```python
from build123d import *

# Parameters (mm, degrees)
F0_W      = 37
F0_H      = 107
F1_DEPTH  = 1.5
F2_W      = 37
F2_H      = 107
F2_W_2    = 33
F2_H_2    = 103
F3_DEPTH  = 15
F4_W      = 7
F4_H      = 7
F5_DEPTH  = 5
F6_R      = 1.5
F7_DEPTH  = 5
F8_R      = 3
F9_W      = 8
F9_H      = 11.456422
F10_DEPTH = 25
F11_W     = 12
F11_H     = 3
F11_H_2   = 4
F11_W_2   = 10
F11_H_3   = 12.768078
F12_DEPTH = 25
F13_R     = 3


with BuildPart() as f1:
    # F0 (on Top) → F1 (new body)
    with BuildSketch(Plane.XY):
        Rectangle(F0_W, F0_H)
    extrude(amount=F1_DEPTH)

    # F2 (on face) → F3 (join)
    with BuildSketch(Plane.XY.offset(1.5)):
        Rectangle(F2_W, F2_H)
        Rectangle(F2_W_2, F2_H_2, mode=Mode.SUBTRACT)
    extrude(amount=F3_DEPTH)

    # F4 (on face) → F5 (join)
    with BuildSketch(Plane.XY.offset(1.5)):
        with Locations((-13, 48)):
            Rectangle(F4_W, F4_H)
        with Locations((13, 48)):
            Rectangle(F4_W, F4_H)
        with Locations((13, -48)):
            Rectangle(F4_W, F4_H)
        with Locations((-13, -48)):
            Rectangle(F4_W, F4_H)
    extrude(amount=F5_DEPTH)

    # F6 (on face) → F7 (cut)
    with BuildSketch(Plane.XY.offset(6.5)):
        with Locations((-12.5, 47.5)):
            Circle(F6_R)
        with Locations((12.5, 47.5)):
            Circle(F6_R)
        with Locations((12.5, -47.5)):
            Circle(F6_R)
        with Locations((-12.5, -47.5)):
            Circle(F6_R)
    extrude(amount=-F7_DEPTH, mode=Mode.SUBTRACT)

    # F8
    f8_edges = [f1.edges().sort_by_distance(p)[0] for p in [
        (-9.5, 44.5, 4),
        (9.5, 44.5, 4),
        (-9.5, -44.5, 4),
        (9.5, -44.5, 4),
    ]]
    fillet(f8_edges, radius=F8_R)

    # F9 (on face) → F10 (cut)
    with BuildSketch(Plane(origin=(0, -51.5, 0), x_dir=(-1, 0, 0), z_dir=(0, 1, 0))):
        with Locations((4, 12.228211)):
            Rectangle(F9_W, F9_H)
        with Locations((-4, 12.228211)):
            Rectangle(F9_W, F9_H)
    extrude(amount=-F10_DEPTH, mode=Mode.SUBTRACT)

    # F11 (on face) → F12 (cut)
    with BuildSketch(Plane(origin=(-18.5, 0, 0), x_dir=(0, -1, 0), z_dir=(-1, 0, 0))):
        with Locations((-39.5, 8)):
            Rectangle(F11_W, F11_H)
        with Locations((-39.5, 4.5)):
            Rectangle(F11_W, F11_H_2)
        with Locations((37.5, 12.884039)):
            Rectangle(F11_W_2, F11_H_3)
    extrude(amount=-F12_DEPTH, mode=Mode.SUBTRACT)

    # F13
    f13_edges = [f1.edges().sort_by_distance(p)[0] for p in [
        (18.5, -53.5, 8.25),
        (-18.5, -53.5, 8.25),
        (-18.5, 53.5, 8.25),
        (18.5, 53.5, 8.25),
    ]]
    fillet(f13_edges, radius=F13_R)


solid = f1.part
```
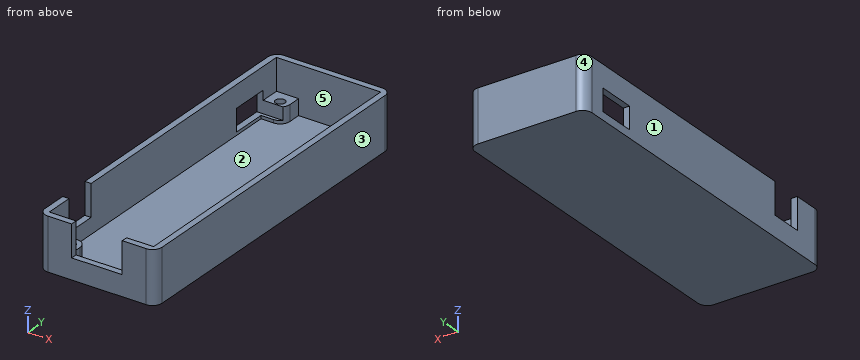
The listing builds one solid part. Answer for the finished solid, in the listing's coordinates (mm). Face numbers are marked on the shaded views. A direction names the side the tool comes from. Round coordinates to 2 decimals unless told otherwise and drop trailing zeros. Write each loop counter-clockwise with the first axis right and the second up, starting at its lowest first coordinate (ties: lowest second). Pieces come first, ordered by that corner, then holes. Notation, with made-up numbers: (-10, 13.5) -> (10, 13.5) arc R18 ccw to (10, 25.5) -> close; hole circle Ø7 at (-37.75, 73.25). An arc over 180 degrees is marked (long way). Answer as a JSON object with one key per item and string values. Group by question number.
Q1. Each of these flat-tipped pins is pushed along its axis until it touches: pin 1 Ø2 at (x, z) = (-18, 9.5) entering from +Y; pin 2 Ø6 at (x, y) = (3, -28.5) entering from +Z; pin 3 Ø6.5 at (x, y) = (-12, 47) entering from +Z. Where does it stop, or does it pass through?
Q2. Section A-A (y = 36) is taken. Write down the section's boundary in (x, z), plus the area to 4 significant figures.
Q3. Which of the six approach directions +Z, -Z, +X, -X, +Y, -Y give full straight-line access (tool end or side, diameter ignored) to the marked faces 4 and 5?
Q4. Straight lines are drawn through the part: line 1 along Y through (x, z) = (-12.5, 2.7); line 2 along Y through (x, z) = (12.5, 3.65); line 3 along X through (y, z) = (41.5, 15.75). For each, find the intervals that lie inside material, in ascending order.
Q5. Section C-C (y = 2.5) is taken. Write down the section's boundary in (x, z).
Q6. Section B-B (z = 12.75) is taken. Write down the section's boundary in (x, y).
Q7. Determine the mould class of the marked faces 1, 2 and 3 for opening direction X: pulls with the +X half, pulls with the -X half, needs draft (parallel to the pull), parting line crosses it, or undercut.
Check values:
{
 "1": {"pin 1": "y = 53.1", "pin 2": "z = 1.5", "pin 3": "z = 6.5"},
 "2": {"outline": "(-18.5, 0) -> (18.5, 0) -> (18.5, 16.5) -> (16.5, 16.5) -> (16.5, 1.5) -> (-16.5, 1.5) -> (-16.5, 2.5) -> (-18.5, 2.5) -> close; (-18.5, 9.5) -> (-16.5, 9.5) -> (-16.5, 16.5) -> (-18.5, 16.5) -> close", "area": "101.5 mm^2"},
 "3": {"face 4": "+Z, -Z, -X, +Y", "face 5": "+Z"},
 "4": {"line 1": "-53.5 to -49, -46 to -44.5, 45.5 to 46, 49 to 53.5", "line 2": "-53.5 to -49, -46 to -44.5, 44.5 to 46, 49 to 53.5", "line 3": "-18.5 to -16.5, 16.5 to 18.5"},
 "5": {"outline": "(-18.5, 0) -> (18.5, 0) -> (18.5, 16.5) -> (16.5, 16.5) -> (16.5, 1.5) -> (-16.5, 1.5) -> (-16.5, 16.5) -> (-18.5, 16.5) -> close"},
 "6": {"outline": "(-18.5, -50.5) arc R3 ccw to (-15.5, -53.5) -> (-8, -53.5) -> (-8, -51.5) -> (-16.5, -51.5) -> (-16.5, -42.5) -> (-18.5, -42.5) -> close; (-18.5, -32.5) -> (-16.5, -32.5) -> (-16.5, 51.5) -> (16.5, 51.5) -> (16.5, -51.5) -> (8, -51.5) -> (8, -53.5) -> (15.5, -53.5) arc R3 ccw to (18.5, -50.5) -> (18.5, 50.5) arc R3 ccw to (15.5, 53.5) -> (-15.5, 53.5) arc R3 ccw to (-18.5, 50.5) -> close"},
 "7": {"face 1": "pulls with the -X half", "face 2": "undercut", "face 3": "pulls with the +X half"}
}
